```python
from build123d import *

# Parameters (mm, degrees)
F0_R     = 13.75
F0_R_2   = 1.5
F1_DEPTH = 18.34
F2_R     = 5
F3_DEPTH = 1
F4_R     = 0.8
F5_DEPTH = 15


# Not quite as in the source:
# - a fillet or chamfer that OpenCascade refuses, or shapes differently, is made with other operations: its cross-section is extruded or revolved along the edge and cut away or added


with BuildPart() as f1:
    # F0 (on Front) → F1 (new body)
    with BuildSketch(Plane.XZ):
        Circle(F0_R)
        with Locations((0, -8)):
            Circle(F0_R_2, mode=Mode.SUBTRACT)
        with Locations((-9.5, 0)):
            Circle(F0_R_2, mode=Mode.SUBTRACT)
        with Locations((9.5, 0)):
            Circle(F0_R_2, mode=Mode.SUBTRACT)
        with Locations((0, 8)):
            Circle(F0_R_2, mode=Mode.SUBTRACT)
    extrude(amount=F1_DEPTH)

    # F2 (on Front) → F3 (join)
    with BuildSketch(Plane.XZ):
        Circle(F2_R)
    extrude(amount=-F3_DEPTH)

    # F4 (on Front) → F5 (join)
    with BuildSketch(Plane.XZ):
        Circle(F4_R)
    extrude(amount=-F5_DEPTH)

    # F6: fillet of radius 3 on 1 edges, made by hand

    # F6_s1 → F6_t2 (revolve, cut)
    with BuildSketch(Plane.XY):
        with BuildLine():
            ThreePointArc((13.75, -3), (12.8713203436, -0.8786796564), (10.75, 0))
            Line((10.75, 0), (13.75, 0))
            Line((13.75, 0), (13.75, -3))
        make_face()
    revolve(axis=Axis((0, 0, 0), (0, -1, 0)), mode=Mode.SUBTRACT)


solid = f1.part
```
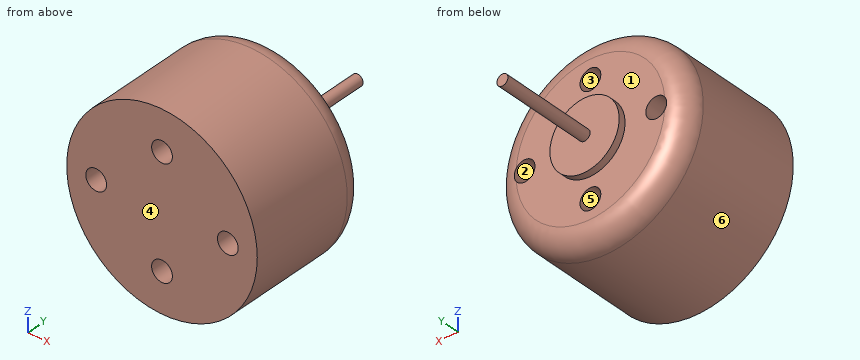
Verification items for the finished model (mm, model axes). Face numbers are marked on the shaded views. A direction names the side the tool comes from. Round coordinates to 2 decimals unless told otherwise and drop trailing zeros. Write each loop counter-clockwise with the first axis right and the second up, starting at its lowest first coordinate (ties: lowest second). Pieces come first, ordered by that corner, then holes.
1. Draft check along Z on the marked faces 3, 4, 5 and 6. Enter one of: +Z half, -Z half, draft (parallel to the pull), parting line (faces both ways), or undercut.
2. Access from +Z, -Z, +X, -X, +Y, -Y to the whole of each face (thin tool, end or side, straight path). Record for the marked faces 1 and 2.
3. Section check C-C on y = 8. Enter the section's corners in (x, z).
4. Section check B-B on y = -9. Enter the section's corners in (x, z), plus the area to 3 significant figures.
5. Gauge pin test, flat ends, axial feed: P1, Ø5, axis at x = -1, z = 5.5, coming from the +Y side; P2, Ø1.5, axis at y = -2, z = -5, coming from the -X side; P3, Ø4, axis at y = -10.5, z = -5.5, coming from the -X side; P4, Ø1.8, axis at x = -9.5, z = 0, coming from the -Y side. Record the tip position at first contact, or that the pin passes through.
6. Section check A-A on x = 0. Enter the section's corners in (y, z).
7. Scan lines: L1, parallel to Z at x = 0, y = -6; L2, parallel to Y at x = 8, z = 3.25; L3, parallel to Z at x = -9.5, y = -14. Record each from-to range of solid material in increasing order.
Answer:
1. face 3: undercut
1. face 4: draft
1. face 5: undercut
1. face 6: parting line
2. face 1: +Y
2. face 2: +Y, -Y
3. outline: circle Ø1.6 at (0, 0)
4. outline: circle Ø27.5 at (0, 0); hole circle Ø3 at (-9.5, 0); hole circle Ø3 at (0, -8); hole circle Ø3 at (0, 8); hole circle Ø3 at (9.5, 0)
4. area: 566 mm2
5. P1: stops at y = 1
5. P2: stops at x = -12.97
5. P3: stops at x = -13.3
5. P4: passes through
6. outline: (-18.34, -13.75) - (-3, -13.75) arc R3 ccw to (0, -10.75) - (0, -9.5) - (-18.34, -9.5) - close; (-18.34, -6.5) - (0, -6.5) - (0, -5) - (1, -5) - (1, -0.8) - (15, -0.8) - (15, 0.8) - (1, 0.8) - (1, 5) - (0, 5) - (0, 6.5) - (-18.34, 6.5) - close; (-18.34, 9.5) - (0, 9.5) - (0, 10.75) arc R3 ccw to (-3, 13.75) - (-18.34, 13.75) - close
7. L1: z = -13.75 to -9.5, -6.5 to 6.5, 9.5 to 13.75
7. L2: y = -18.34 to 0
7. L3: z = -9.94 to -1.5, 1.5 to 9.94
